Geometry: final body of the model. Coordinates: model frame, mm. A direction names the side the tool comes from. Coordinates: 2 decimals unless noted, no trailing zeros. Loops run counter-clockwise (first coordinate to the right, second up) from the corner with the lowest first, then second, coordinate; pieces in that order, holes last. Notation, with made-up numbers: M 52.25,22.5 L 56.25,22.5 A30 ccw 56.25,51.5 Z; hole C 85,45 d9. An arc over 180 degrees is marked long. Write each question's results on one line, items separated by ' | '. Start each with the question number.
from build123d import *

# Parameters (mm, degrees)
F0_R      = 17.5
F0_R_2    = 10.75
F1_DEPTH  = 6
F2_R      = 10.75
F2_R_2    = 1.75
F3_DEPTH  = 4
F8_DEPTH  = 6
F9_DEPTH  = 6
F11_DEPTH = 50
F12_R     = 4.75
F13_DEPTH = 1
F14_R     = 3
F15_DEPTH = 1.5


with BuildPart() as f1:
    # F0 (on Top) → F1 (new body)
    with BuildSketch(Plane.XY):
        Circle(F0_R)
        Circle(F0_R_2, mode=Mode.SUBTRACT)
    extrude(amount=F1_DEPTH)

    # F2 (on Top) → F3 (join)
    with BuildSketch(Plane.XY):
        Circle(F2_R)
        Circle(F2_R_2, mode=Mode.SUBTRACT)
    extrude(amount=F3_DEPTH)

    # F5: sweep along a path in F5_path
    with BuildLine(Plane(origin=(17.5, 0, 6), x_dir=(0, -1, 0), z_dir=(0, 0, -1))) as f5_path:
        CenterArc((0, 17.5), 17.5, 0, 360)
    # F4 (on Front) → F5 (sweep, cut)
    with BuildSketch(Plane.XZ):
        Polygon((17.5310889132, 4.75), (14.5, 3), (17.5310889132, 1.25), align=None)
    sweep(path=f5_path.line, mode=Mode.SUBTRACT)

    # F6 (on Top) → F8 (cut)
    with BuildSketch(Plane.XY):
        with BuildLine():
            Line((-4, 8.8917096219), (4, 8.8917096219))
            ThreePointArc((4, 8.8917096219), (0, 9.75), (-4, 8.8917096219))
        make_face()
        with BuildLine():
            ThreePointArc((-4, 8.8917096219), (0, 9.75), (4, 8.8917096219))
            Line((4, 8.8917096219), (9.5, 18.4179890635))
            Line((9.5, 18.4179890635), (-9.5, 18.4179890635))
            Line((-9.5, 18.4179890635), (-4, 8.8917096219))
        make_face()
    extrude(amount=F8_DEPTH, mode=Mode.SUBTRACT)

    # F7 (on Top) → F9 (join)
    with BuildSketch(Plane.XY):
        with BuildLine():
            Line((-5.942998404, 12.2570815767), (-7.8859968081, 15.6224535315))
            ThreePointArc((-7.8859968081, 15.6224535315), (-9.1966080897, 14.8886668189), (-10.4394679259, 14.0451952433))
            Line((-10.4394679259, 14.0451952433), (-8.5410746154, 10.7570815767))
            Line((-8.5410746154, 10.7570815767), (-5.942998404, 12.2570815767))
        make_face()
        with BuildLine():
            Line((5.942998404, 12.2570815767), (4.5023149906, 9.761744707))
            ThreePointArc((4.5023149906, 9.761744707), (5.8218855082, 9.037043163), (7.027274843, 8.1351034585))
            Line((7.027274843, 8.1351034585), (8.5410746154, 10.7570815767))
            Line((8.5410746154, 10.7570815767), (5.942998404, 12.2570815767))
        make_face()
        with BuildLine():
            ThreePointArc((7.027274843, 8.1351034585), (5.8218855082, 9.037043163), (4.5023149906, 9.761744707))
            Line((4.5023149906, 9.761744707), (7.027274843, 8.1351034585))
        make_face()
        with BuildLine():
            Line((-4.5023149906, 9.761744707), (-5.942998404, 12.2570815767))
            Line((-5.942998404, 12.2570815767), (-8.5410746154, 10.7570815767))
            Line((-8.5410746154, 10.7570815767), (-7.027274843, 8.1351034585))
            ThreePointArc((-7.027274843, 8.1351034585), (-5.8218855082, 9.037043163), (-4.5023149906, 9.761744707))
        make_face()
        with BuildLine():
            Line((-7.027274843, 8.1351034585), (-4.5023149906, 9.761744707))
            ThreePointArc((-4.5023149906, 9.761744707), (-5.8218855082, 9.037043163), (-7.027274843, 8.1351034585))
        make_face()
        with BuildLine():
            Line((7.8859968081, 15.6224535315), (5.942998404, 12.2570815767))
            Line((5.942998404, 12.2570815767), (8.5410746154, 10.7570815767))
            Line((8.5410746154, 10.7570815767), (10.4394679259, 14.0451952433))
            ThreePointArc((10.4394679259, 14.0451952433), (9.1966080897, 14.8886668189), (7.8859968081, 15.6224535315))
        make_face()
    extrude(amount=F9_DEPTH)

    # F10 (on Right) → F11 (cut, symmetric)
    with BuildSketch(Plane.YZ):
        with BuildLine():
            ThreePointArc((12, 2.25), (12.5303300859, 2.4696699141), (12.75, 3))
            ThreePointArc((12.75, 3), (11.4696699141, 3.5303300859), (12, 2.25))
        make_face()
    extrude(amount=F11_DEPTH, both=True, mode=Mode.SUBTRACT)

    # F12 (on face) → F13 (cut)
    with BuildSketch(Plane.XY.offset(4)):
        Circle(F12_R)
    extrude(amount=-F13_DEPTH, mode=Mode.SUBTRACT)

    # F14 (on Top) → F15 (cut)
    with BuildSketch(Plane.XY):
        Circle(F14_R)
    extrude(amount=F15_DEPTH, mode=Mode.SUBTRACT)


solid = f1.part
Item 1: Contact query for flat-ended pins moving along their axis: P1, Ø0.9, axis at y = 12, z = 3, coming from the -X side; P2, Ø15, axis at x = 0, y = 0, coming from the +Z side; P3, Ø5.5, axis at x = 0, y = 0, coming from the +Z side; P4, Ø3, axis at x = -1, y = -1, coming from the -Z side. Output: stop coordinate, or through.
Item 2: Section B-B, the plane x = 0. Return loops of the section in (y, z).
Item 3: Pull-direction query (Z, two-part tool) for faces 1 (the flat face through (0, 8.892, 2)), 2 (the flat face through (0, -4, 0)), 3 (the flat face through (0, -5, 4)), 4 (the flat face through (-10.075, 13.414, 2.976)); classes: released by +Z, released by -Z, zero draft, split by the parting line, or undercut.
Item 4: Set-up query: faces 5 (the conical face through (0.51, -14.68, 2.89)), 6 (the flat face through (0, -2, 1.5)), 7 (the flat face through (10.06, 13.39, 2.98)), 8 (the flat face through (2, 0, 3)). Return all of +Z, -Z, +X, -X, +Y, -Y with unobstructed straight access to the full face (end or side cutting, diameter ignored); none if empty.
Item 5: Ray query, L1, parallel to X at y = 0, z = 5.45; L2, parallel to Z at x = 6, y = 12; L3, parallel to Z at x = -2.5, y = 1.5. Return the intervals inside material, ascending. Write a range as [from, to].
Item 6: Section A-A, the plane y = 0. Return loops of the section in (x, z), plus the area to 3 significant figures.
Solutions:
1) P1: passes through | P2: stops at z = 4 | P3: stops at z = 3 | P4: stops at z = 1.5
2) outline: M -17.5,0 L -3,0 L -3,1.5 L -1.75,1.5 L -1.75,3 L -4.75,3 L -4.75,4 L -10.75,4 L -10.75,6 L -17.5,6 L -17.5,4.73 L -14.5,3 L -17.5,1.27 Z; M 1.75,1.5 L 3,1.5 L 3,0 L 8.89,0 L 8.89,4 L 4.75,4 L 4.75,3 L 1.75,3 Z
3) face 1: zero draft | face 2: released by -Z | face 3: released by +Z | face 4: undercut
4) face 5: none | face 6: -Z | face 7: +X | face 8: +Z
5) L1: x = [-17.5, -10.75], [10.75, 17.5] | L2: z = [0, 2.25], [3.75, 6] | L3: z = [1.5, 3]
6) outline: M -17.5,0 L -3,0 L -3,1.5 L -1.75,1.5 L -1.75,3 L -4.75,3 L -4.75,4 L -10.75,4 L -10.75,6 L -17.5,6 L -17.5,4.73 L -14.5,3 L -17.5,1.27 Z; M 1.75,1.5 L 3,1.5 L 3,0 L 17.5,0 L 17.5,1.27 L 14.5,3 L 17.5,4.73 L 17.5,6 L 10.75,6 L 10.75,4 L 4.75,4 L 4.75,3 L 1.75,3 Z | area: 133 mm²
